```python
from build123d import *

# Parameters (mm, degrees)
F1_DEPTH = 200
F2_R     = 5
F3_R     = 6
F4_DEPTH = 25
F6_DEPTH = 25


with BuildPart() as f1:
    # F0 (on Front) → F1 (new body)
    with BuildSketch(Plane.XZ):
        Polygon((0, 90), (0, 0), (90, 0), (90, 12), (12, 12), (12, 90), align=None)
    extrude(amount=F1_DEPTH)

    # F2
    f2_edges = [f1.edges().sort_by_distance(p)[0] for p in [
        (12, -100, 90),
        (12, -100, 12),
        (90, -100, 12),
        (90, -100, 0),
        (0, -100, 90),
        (0, -100, 0),
    ]]
    fillet(f2_edges, radius=F2_R)

    # F3 (on face) → F4 (cut)
    with BuildSketch(Plane.YZ.offset(12)):
        with Locations((-100, 46)):
            Circle(F3_R)
    extrude(amount=-F4_DEPTH, mode=Mode.SUBTRACT)

    # F5 (on face) → F6 (cut)
    with BuildSketch(Plane.XY.offset(12)):
        with BuildLine():
            Line((66, -145.373556), (36, -145.373556))
            ThreePointArc((36, -145.373556), (29.75, -151.623556), (36, -157.873556))
            Line((36, -157.873556), (66, -157.873556))
            ThreePointArc((66, -157.873556), (72.25, -151.623556), (66, -145.373556))
        make_face()
        with BuildLine():
            Line((66, -43.75), (36, -43.75))
            ThreePointArc((36, -43.75), (29.75, -50), (36, -56.25))
            Line((36, -56.25), (66, -56.25))
            ThreePointArc((66, -56.25), (72.25, -50), (66, -43.75))
        make_face()
    extrude(amount=-F6_DEPTH, mode=Mode.SUBTRACT)


solid = f1.part
```
Design review of the part built by this model. Coordinates are the model's own, in mm. A direction names the side the tool comes from. Coordinates: 2 decimals unless noted, no trailing zeros. Order: outer loops, then holes, each group sorted by start corner. A loop starts at its lowest first (then second) coordinate and runs counter-clockwise, first axis right, second up.
1) Take a section at D-D, the plane y = -135.5. Give the boundary of the cut face in (x, z).
2) Take a section at B-B, the plane x = 55.5. Give the boundary of the cut face in (y, z), and give its area (3 significant figures).
3) Clearance check with flat-ended pins moving along their axes: pin 1 (3.5 mm diameter, centred on x = 45, z = 4, fed in from +Y); pin 2 (2 mm diameter, centred on x = 53.5, y = -67.5, fed in from +Z); pin 3 (6 mm diameter, centred on y = -85.5, z = 70.5, fed in from +X). State where each tip first meets the part, or that it passes through.
4) Wall thickness on line 1 along Z through (x, y) = (6.5, -100); line 2 along Z through (x, y) = (84.5, -132): over which ranges is each line inside the solid? List them lowest first.
5) For faces 5 (the flat face through (51, -99, 12)), 6 (the flat face through (51, -56.25, 6)), 7 (the flat face through (11, 0, 29)), list the 3-axis set-ups (+Z, -Z, +X, -X, +Y, -Y) from which the entire face can be reached by the end or side of a thin tool; tool diameter is ignored.
6) Take a section at C-C, the plane z = 46. Give the boundary of the cut face in (x, y).
7) Mouldability with a two-part tool opening along X and no side actions: class faces 1 (the flat face through (51, -43.75, 6)), 2 (the flat face through (11, -200, 29)), 3 (the cylindrical face through (1, -101, 2)), 4 (the cylindrical face through (11, -101, 88)) as +X half, -X half, draft (parallel to the pull), parting line (faces both ways), or undercut.
8) Take a section at A-A, the plane y = -100. Give the boundary of the cut face in (x, z).
Returned:
1. outline: (0, 5) arc R5 ccw to (5, 0) - (85, 0) arc R5 ccw to (90, 5) - (90, 7) arc R5 ccw to (85, 12) - (17, 12) arc R5 cw to (12, 17) - (12, 85) arc R5 ccw to (7, 90) - (5, 90) arc R5 ccw to (0, 85) - close
2. outline: (-200, 0) - (-157.87, 0) - (-157.87, 12) - (-200, 12) - close; (-145.37, 0) - (-56.25, 0) - (-56.25, 12) - (-145.37, 12) - close; (-43.75, 0) - (0, 0) - (0, 12) - (-43.75, 12) - close
2. area: 2,100 mm2
3. pin 1: stops at y = 0
3. pin 2: stops at z = 12
3. pin 3: stops at x = 12
4. line 1: z = 0 to 40, 52 to 90
4. line 2: z = 0 to 12
5. face 5: +Z, +X, +Y, -Y
5. face 6: +Z, -Z
5. face 7: +Z, -Z, +X, -X, +Y
6. outline: (0, -200) - (12, -200) - (12, -106) - (0, -106) - close; (0, -94) - (12, -94) - (12, 0) - (0, 0) - close
7. face 1: undercut
7. face 2: draft
7. face 3: -X half
7. face 4: +X half
8. outline: (0, 5) arc R5 ccw to (5, 0) - (85, 0) arc R5 ccw to (90, 5) - (90, 7) arc R5 ccw to (85, 12) - (17, 12) arc R5 cw to (12, 17) - (12, 40) - (0, 40) - close; (0, 52) - (12, 52) - (12, 85) arc R5 ccw to (7, 90) - (5, 90) arc R5 ccw to (0, 85) - close
